from build123d import *

# Parameters (mm, degrees)
SKETCH1_R           = 25
BOSS_EXTRUDE1_DEPTH = 8.5
SKETCH2_R           = 6
SKETCH2_R_2         = 2.5
BOSS_EXTRUDE2_DEPTH = 10


with BuildPart() as part:
    # Sketch1 → Boss-Extrude1 (new body)
    with BuildSketch(Plane.XY):
        Circle(SKETCH1_R)
    extrude(amount=BOSS_EXTRUDE1_DEPTH)

    # Sketch2 → Boss-Extrude2 (add)
    with BuildSketch(Plane(origin=(0, 0, 0), x_dir=(-1, 0, 0), z_dir=(0, 0, -1))):
        Circle(SKETCH2_R)
        Circle(SKETCH2_R_2, mode=Mode.SUBTRACT)
    extrude(amount=BOSS_EXTRUDE2_DEPTH)


solid = part.part
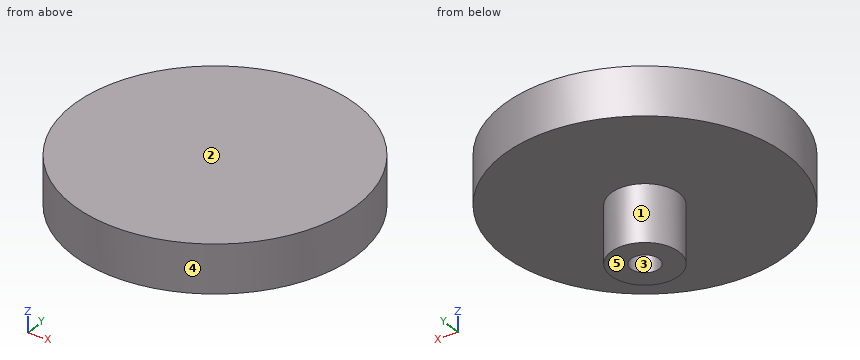
Read the model definition and answer for the solid it produces. Units are mm, in the model's axes. Face numbers are marked on the shaded views. A direction names the side the tool comes from. Round coordinates to 2 decimals unless told otherwise and drop trailing zeros. Write each loop counter-clockwise with the first axis right and the second up, starting at its lowest first coordinate (ties: lowest second). Pieces come first, ordered by that corner, then holes. Notation, with made-up numbers: M 9,64.25 L 25,64.25 A21 cw 25,76.25 Z; hole C 57.25,10 d6. An arc over 180 degrees is marked long. Use a Markdown table: item, result.
1) For a pull along X with two mould halves and no side action, classify the marked faces 3, 4 and 5 as pulls with the +X half, pulls with the -X half, needs draft (parallel to the pull), parting line crosses it, or undercut.
Answers follow:
| item | result |
|---|---|
| face 3 | undercut |
| face 4 | parting line crosses it |
| face 5 | needs draft |
2) Flat-ended cylindrical pins translate along their axes: pin 1 (2 mm diameter, centred on y = 6, z = -5.5, fed in from -X); pin 2 (2 mm diameter, centred on x = 16.5, z = 6, fed in from +Y); pin 3 (1 mm diameter, centred on y = 3.5, z = -1, fed in from +X); pin 4 (5 mm diameter, centred on x = 15, z = -4.5, fed in from -Y). Find the tip coordinate at first contact, or state that the pin passes through.
Answers follow:
| item | result |
|---|---|
| pin 1 | stops at x = -3.32 |
| pin 2 | stops at y = 19.62 |
| pin 3 | stops at x = 5.2 |
| pin 4 | passes through |
3) The part is cut by section D-D (y = -5). Write down the section's boundary in (x, z).
Answers follow:
| item | result |
|---|---|
| outline | M -24.49,0 L -3.32,0 L -3.32,-10 L 3.32,-10 L 3.32,0 L 24.49,0 L 24.49,8.5 L -24.49,8.5 Z |
4) A tool of negligible diameter and unlimited length cuts with its end or side. For the marked faces 1 and 2, from which of +Z, -Z, +X, -X, +Y, -Y can it reach the whole face along a straight path? Write none if from no direction.
Answers follow:
| item | result |
|---|---|
| face 1 | -Z |
| face 2 | +Z, +X, -X, +Y, -Y |
5) Straight lines are drawn through the part: line 1 along Y through (x, z) = (0, -7); line 2 along Z through (x, y) = (10.5, 1); line 3 along X through (y, z) = (-7, 4.5). For each, find the intervals that lie inside material, in ascending order. Write a range as [from, to].
Answers follow:
| item | result |
|---|---|
| line 1 | y = [-6, -2.5], [2.5, 6] |
| line 2 | z = [0, 8.5] |
| line 3 | x = [-24, 24] |
6) The part is cut by section C-C (z = -7). Write down the section's boundary in (x, y).
Answers follow:
| item | result |
|---|---|
| outline | C 0,0 d12; hole C 0,0 d5 |
7) The part is cut by section A-A (x = 0). Write down the section's boundary in (y, z), plus the area to 3 significant figures.
Answers follow:
| item | result |
|---|---|
| outline | M -25,0 L -6,0 L -6,-10 L -2.5,-10 L -2.5,0 L 2.5,0 L 2.5,-10 L 6,-10 L 6,0 L 25,0 L 25,8.5 L -25,8.5 Z |
| area | 495 mm2 |
